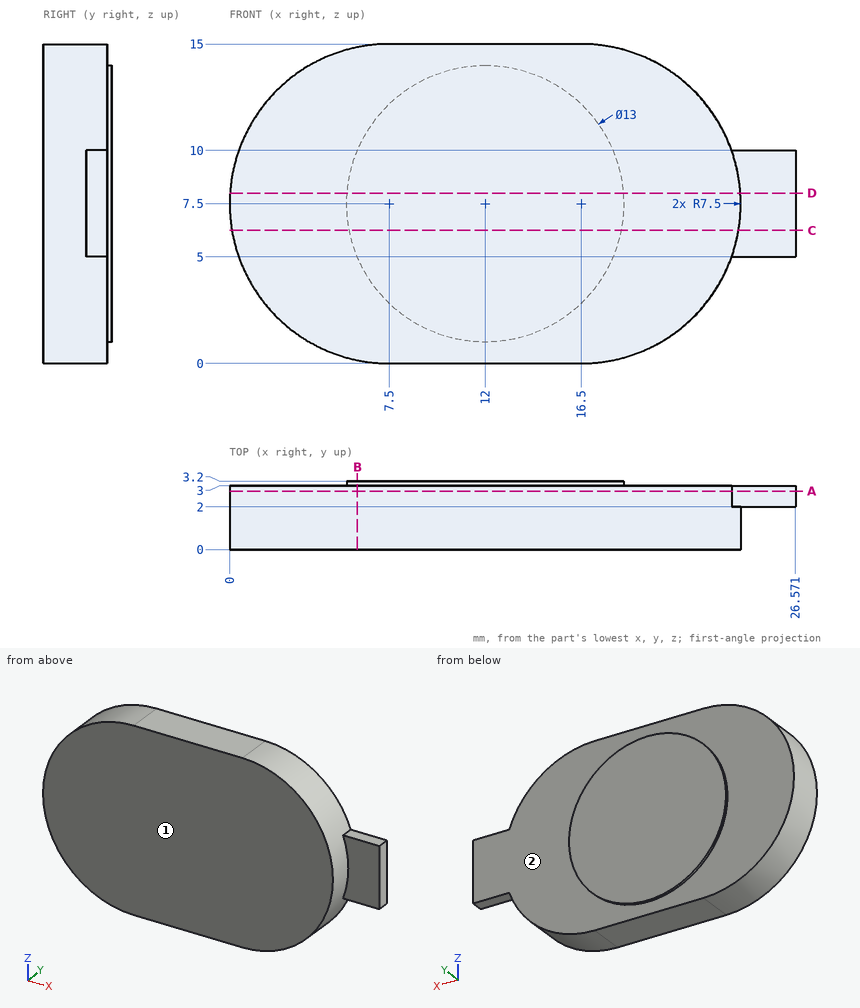
Here's the drawing with two shaded views (mm, measured from the low corner). I have some questions. A direction names the side the tool comes from. Coordinates: 2 decimals unless noted, no trailing zeros. Write each loop counter-clockwise with the first axis right and the second up, starting at its lowest first coordinate (ties: lowest second). Pieces come first, ordered by that corner, then holes. Notation, with made-up numbers: (35, -20.5) -> (64, -20.5) arc R25 ccw to (64, 17.5) -> close; hole circle Ø8 at (-21, -18). An arc over 180 degrees is marked (long way). One line per question, with ' | ' between items. Start each with the question number.
1. If we section it at A-A (y = 2.75): Please give me the cut outline in (x, z).
2. If we section it at B-B (x = 6): Please give me the cut outline in (y, z), and give its area (3 significant figures).
3. If we section it at D-D (z = 8): Please give me the cut outline in (x, y).
4. If we section it at C-C (z = 6.25): Please give me the cut outline in (x, y) (3 decimals).
5. For the marked faces 1 and 2, which set-ups out of +Z, -Z, +X, -X, +Y, -Y let a thin tool reach every point of the face, with its end or its side?
6. Will these pins go through, and if not, where does the flat tip stop? P1, Ø8, axis at x = 2.5, z = 12.5, coming from the +Y side; P2, Ø0.8, axis at x = 24.5, y = 2.5, coming from the -Z side; P3, Ø1.1, axis at x = 24.5, y = 2.5, coming from the +Z side.
7. Please list where these lines run through material, in increasing order: line 1 along Y through (x, z) = (2.5, 3); line 2 along Y through (x, z) = (25, 6.25); line 3 along Z through (x, y) = (2.5, 1.55).
Return value:
1) outline: (7.5, 0) -> (16.5, 0) arc R7.5 ccw to (23.57, 5) -> (26.57, 5) -> (26.57, 10) -> (23.57, 10) arc R7.5 ccw to (16.5, 15) -> (7.5, 15) arc R7.5 ccw to start
2) outline: (0, 0.15) -> (3, 0.15) -> (3, 5) -> (3.2, 5) -> (3.2, 10) -> (3, 10) -> (3, 14.85) -> (0, 14.85) -> close | area: 45.1 mm²
3) outline: (0.02, 0) -> (23.98, 0) -> (23.98, 2) -> (26.57, 2) -> (26.57, 3) -> (18.48, 3) -> (18.48, 3.2) -> (5.52, 3.2) -> (5.52, 3) -> (0.02, 3) -> close
4) outline: (0.105, 0) -> (23.895, 0) -> (23.895, 2) -> (26.571, 2) -> (26.571, 3) -> (18.379, 3) -> (18.379, 3.2) -> (5.621, 3.2) -> (5.621, 3) -> (0.105, 3) -> close
5) face 1: +Z, -Z, +X, -X, -Y | face 2: +Y
6) P1: stops at y = 3 | P2: stops at z = 5 | P3: stops at z = 10
7) line 1: y = 0 to 3 | line 2: y = 2 to 3 | line 3: z = 1.91 to 13.09
